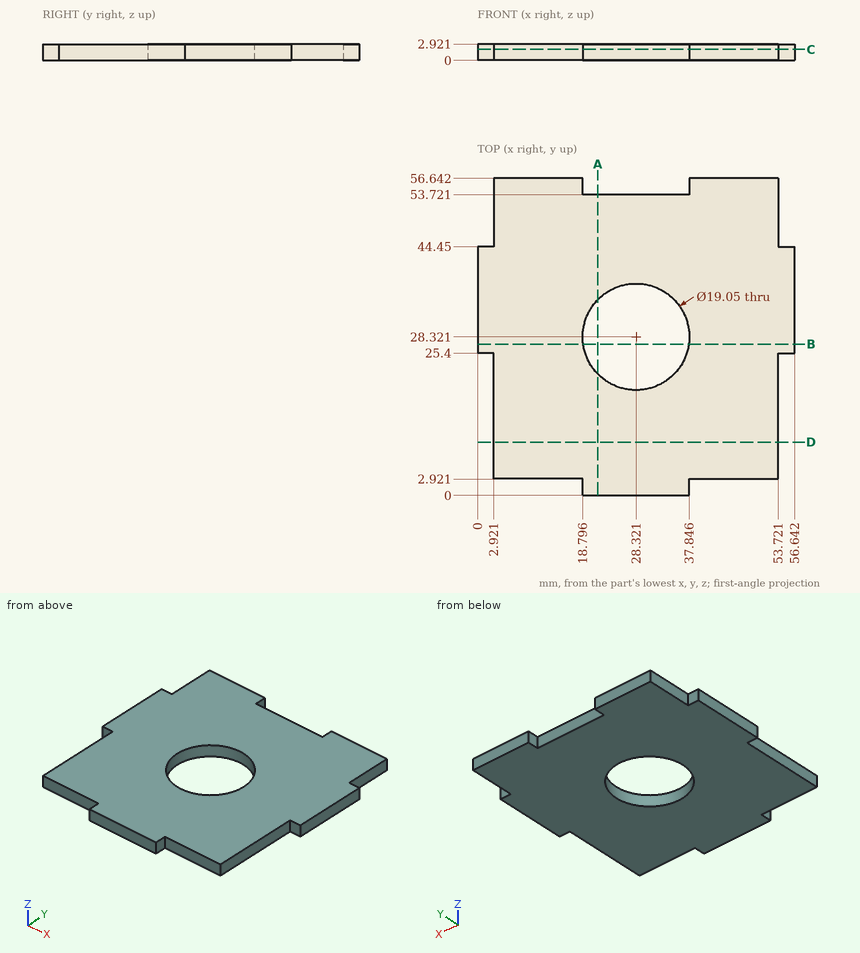
Here's the drawing with two shaded views (mm, measured from the low corner). I have some questions. Give positions to 0.01 mm unless a question says otherwise; leave off trailing zeros. Write each loop counter-clockwise with the first axis right and the second up, starting at its lowest first coordinate (ties: lowest second). Pieces come first, ordered by that corner, then holes. Notation, with made-up numbers: (17, -31) -> (29, -31) arc R12 ccw to (29, -21) -> close; hole circle Ø5 at (-39.5, 60). An arc over 180 degrees is marked (long way). Use one line per item in the form item = value.
1) I'm going to push flat-ended pins straight in: pin 1 (0.9 mm diameter, centred on y = 49, z = 1, fed in from +X); pin 2 (0.9 mm diameter, centred on x = 32, z = 2, fed in from +Y); pin 3 (1.5 mm diameter, centred on x = 12, z = 2, fed in from -Y). Where does each tip first touch, or does it pass through?
Verdict:
pin_1 = 53.72
pin_2 = 53.72
pin_3 = 2.92
2) Suppose I cut it at C-C (z = 1.95). Please give me the cut outline in (x, y) (3 decimals), and give its area (3 significant figures).
Verdict:
outline = (0, 25.4) -> (2.921, 25.4) -> (2.921, 2.921) -> (18.796, 2.921) -> (18.796, 0) -> (37.846, 0) -> (37.846, 2.921) -> (53.721, 2.921) -> (53.721, 25.4) -> (56.642, 25.4) -> (56.642, 44.45) -> (53.721, 44.45) -> (53.721, 56.642) -> (37.846, 56.642) -> (37.846, 53.721) -> (18.796, 53.721) -> (18.796, 56.642) -> (2.921, 56.642) -> (2.921, 44.45) -> (0, 44.45) -> close; hole circle Ø19.05 at (28.321, 28.321)
area = 2,560 mm2
3) Suppose I cut it at D-D (y = 9.5). Please give me the cut outline in (x, z), and give its area (3 significant figures).
Verdict:
outline = (2.92, 0) -> (53.72, 0) -> (53.72, 2.92) -> (2.92, 2.92) -> close
area = 148 mm2
4) Suppose I cut it at A-A (x = 21.5). Please give me the cut outline in (y, z).
Verdict:
outline = (0, 0) -> (21.67, 0) -> (21.67, 2.92) -> (0, 2.92) -> close; (34.97, 0) -> (53.72, 0) -> (53.72, 2.92) -> (34.97, 2.92) -> close
5) Suppose I cut it at B-B (y = 27). Please give me the cut outline in (x, z), and give its area (3 significant figures).
Verdict:
outline = (0, 0) -> (18.89, 0) -> (18.89, 2.92) -> (0, 2.92) -> close; (37.75, 0) -> (56.64, 0) -> (56.64, 2.92) -> (37.75, 2.92) -> close
area = 110 mm2
6) If I drill on L1, parallel to Y at x = 28.5, z = 0.8; L2, parallel to X at y = 53, z = 2.1; L3, parallel to Y at x = 30, z = 0.7, over which ranges is the centre line in solid material (lowest first)? Write a range as [from, to].
Verdict:
L1 = [0, 18.8], [37.84, 53.72]
L2 = [2.92, 53.72]
L3 = [0, 18.95], [37.7, 53.72]
